Geometry check sheet. Reference: the model listing, model coordinates, mm. A direction names the side the tool comes from. Coordinates: 2 decimals unless noted, no trailing zeros. Write each loop counter-clockwise with the first axis right and the second up, starting at its lowest first coordinate (ties: lowest second). Pieces come first, ordered by that corner, then holes.
Autodesk Inventor part; units mm, degrees
ref_plane "YZ Plane" through (0, 0, 0) normal (1, 0, 0) x (0, 1, 0)
ref_plane "XZ Plane" through (0, 0, 0) normal (0, 1, 0) x (-1, 0, 0)
ref_plane "XY Plane" through (0, 0, 0) normal (0, 0, 1) x (1, 0, 0)
sketch "Sketch1" plane through (0, 0, 0) normal (0, 0, 1) x (1, 0, 0)
  line L0 (0, 0) -> (50.8, 0)
  line L1 (50.8, 0) -> (50.8, -3.175)
  line L2 (50.8, -3.175) -> (3.175, -3.175)
  line L3 (3.175, -3.175) -> (3.175, -25.4)
  line L4 (3.175, -25.4) -> (0, -25.4)
  line L5 (0, -25.4) -> (0, 0)
  dimension "d0" = 3.175
  dimension "d1" = 50.8
  dimension "d2" = 25.4
extrude "Extrusion1" add sketch "Sketch1" along normal blind 177.8
hole "Hole1" at (38.1, 0, 152.4) direction (0, -1, 0) diameter 6.731 depth 25.4 tip angle 118
pattern_linear "Rectangular Pattern1" count 2 spacing 127 along (0, 0, -1) of "Hole1"
properties part number "GE-12028-06"
1. Sectioned sample at D-D, the plane z = 57. Record the boundary of the cut face in (x, y) (3 decimals).
Computed values:
outline: (0, -25.4) - (3.175, -25.4) - (3.175, -3.175) - (50.8, -3.175) - (50.8, 0) - (0, 0) - close
2. Sectioned sample at A-A, the plane z = 25.4. Record the boundary of the cut face in (x, y) (1 decimal), and give its area (3 significant figures).
Computed values:
outline: (0, -25.4) - (3.2, -25.4) - (3.2, -3.2) - (34.7, -3.2) - (34.7, 0) - (0, 0) - close; (41.5, -3.2) - (50.8, -3.2) - (50.8, 0) - (41.5, 0) - close
area: 210 mm2
3. Sectioned sample at B-B, the plane x = 38.1. Record the boundary of the cut face in (y, z) (1 decimal), and give its area (3 significant figures).
Computed values:
outline: (-3.2, 0) - (0, 0) - (0, 22) - (-3.2, 22) - close; (-3.2, 28.8) - (0, 28.8) - (0, 149) - (-3.2, 149) - close; (-3.2, 155.8) - (0, 155.8) - (0, 177.8) - (-3.2, 177.8) - close
area: 522 mm2
4. Thickness scan on line 1 along Z through (x, y) = (38.1, -0.65); line 2 along X through (y, z) = (-1, 25.4); line 3 along Z through (x, y) = (37, -2.75). Record the ranges inside material, lowest first.
Computed values:
line 1: z = 0 to 22.03, 28.77 to 149.03, 155.77 to 177.8
line 2: x = 0 to 34.73, 41.47 to 50.8
line 3: z = 0 to 22.22, 28.58 to 149.22, 155.58 to 177.8
5. Draft check along Z on faces 3 (the flat face through (50.8, -2, 88)), 4 (the cylindrical face through (35.262, -1.61, 27.209)), 5 (the cylindrical face through (37.09, -1.61, 155.61)), 6 (the flat face through (14, -2, 177.8)). Enter one of: released by +Z, released by -Z, zero draft, split by the parting line, or undercut.
Computed values:
face 3: zero draft
face 4: undercut
face 5: undercut
face 6: released by +Z
6. Sectioned sample at C-C, the plane x = 6.5. Record the boundary of the cut face in (y, z) (3 decimals), and give its area (3 significant figures).
Computed values:
outline: (-3.175, 0) - (0, 0) - (0, 177.8) - (-3.175, 177.8) - close
area: 565 mm2
7. Gauge pin test, flat ends, axial feed: pin 1 Ø6 at (x, z) = (38.1, 25.4) entering from +Y; pin 2 Ø11 at (x, z) = (38.1, 152.4) entering from -Y (3 decimals); pin 3 Ø11 at (y, z) = (-15, 124.5) entering from +X (3 decimals). Record the tip position at first contact, or that the pin passes through.
Computed values:
pin 1: passes through
pin 2: stops at y = -3.175
pin 3: stops at x = 3.175
8. Access from +Z, -Z, +X, -X, +Y, -Y to the whole of each face (thin tool, end or side, straight path). Record for faces 1 (the flat face through (25, 0, 88)), 2 (the flat face through (27, -3.175, 88)).
Computed values:
face 1: +Z, -Z, +X, -X, +Y
face 2: +Z, -Z, +X, -Y
